For this review, take the finished solid that the model builds, in its own axes (mm). A direction names the side the tool comes from. Give positions to 0.01 mm unless a question says otherwise; leave off trailing zeros. Write each loop counter-clockwise with the first axis right and the second up, starting at its lowest first coordinate (ties: lowest second). Pieces come first, ordered by that corner, then holes.
from build123d import *

# Parameters (mm, degrees)
F0_W     = 108
F0_H     = 16
F1_DEPTH = 3
F3_D     = 2.4
F3_DEPTH = 6
F3_TIP   = 0.7210327428
F5_D     = 2.4
F5_DEPTH = 6
F5_TIP   = 0.7210327428


with BuildPart() as f1:
    # F0 (on Front) → F1 (new body, symmetric)
    with BuildSketch(Plane.XZ):
        Rectangle(F0_W, F0_H)
        with BuildLine():
            ThreePointArc((-39, -2), (-37, -4), (-39, -6))
            Line((-39, -6), (-48, -6))
            ThreePointArc((-48, -6), (-50, -4), (-48, -2))
            Line((-48, -2), (-39, -2))
        make_face(mode=Mode.SUBTRACT)
        with BuildLine():
            ThreePointArc((-39, 6), (-37, 4), (-39, 2))
            Line((-39, 2), (-48, 2))
            ThreePointArc((-48, 2), (-50, 4), (-48, 6))
            Line((-48, 6), (-39, 6))
        make_face(mode=Mode.SUBTRACT)
    extrude(amount=F1_DEPTH, both=True)

    # F3
    with Locations(Plane(origin=(0, 0, -8), x_dir=(1, 0, 0), z_dir=(0, 0, -1))):
        with Locations((36, 0), (42, 0)):
            Hole(F3_D / 2, depth=F3_DEPTH)
            with Locations((0, 0, -(F3_DEPTH + F3_TIP / 2))):  # 118° drill point
                Cone(0, F3_D / 2, F3_TIP, mode=Mode.SUBTRACT)

    # F5
    with Locations(Plane.XY.offset(8)):
        with Locations((36, 0), (42, 0)):
            Hole(F5_D / 2, depth=F5_DEPTH)
            with Locations((0, 0, -(F5_DEPTH + F5_TIP / 2))):  # 118° drill point
                Cone(0, F5_D / 2, F5_TIP, mode=Mode.SUBTRACT)


solid = f1.part
(1) The part is to be moulded in two halves that separate along Z. For faces 1 (the cylindrical face through (34.89, -0.46, 4.96)), 2 (the flat face through (-1, 0, -8)), 3 (the flat face through (-43, 0, -6)), say which applies: +Z half, -Z half, draft (parallel to the pull), parting line (faces both ways), or undercut.
(2) For L1, parallel to Y at x = 36, z = -4.65; L2, parallel to Z at x = -38, y = -0.35; L3, parallel to X at y = -2.1, z = -3.75, list the stretches that pass through material, from the lowest coordinate up.
(3) Tool access review of faces 4 (the flat face through (54, 0, 0)), 5 (the cylindrical face through (-50, 0, -4)), 6 (the cylindrical face through (40.89, 0.46, -4.96)): name each direction out of +Z, -Z, +X, -X, +Y, -Y from which nothing blocks a thin tool from reaching the whole face with its end or side.
(4) Clearance check with flat-ended pins moving along their axes: pin 1 Ø3 at (x, y) = (42, 0) entering from +Z; pin 2 Ø1.4 at (x, y) = (42, 0) entering from +Z. State where each tip first meets the part, or that it passes through.
(5) We need section B-B (x = -41). Write out the cut boundary in (y, z), and give its area (3 significant figures).
(6) We need section A-A (z = -4). Write out the cut boundary in (x, y).
The answers:
1. face 1: draft
1. face 2: -Z half
1. face 3: undercut
2. L1: y = -3 to -1.2, 1.2 to 3
2. L2: z = -8 to -5.73, -2.27 to 2.27, 5.73 to 8
2. L3: x = -54 to -49.98, -37.02 to 54
3. face 4: +Z, -Z, +X, +Y, -Y
3. face 5: +Y, -Y
3. face 6: -Z
4. pin 1: stops at z = 8
4. pin 2: stops at z = 1.7
5. outline: (-3, -8) - (3, -8) - (3, -6) - (-3, -6) - close; (-3, -2) - (3, -2) - (3, 2) - (-3, 2) - close; (-3, 6) - (3, 6) - (3, 8) - (-3, 8) - close
5. area: 48.0 mm2
6. outline: (-54, -3) - (-50, -3) - (-50, 3) - (-54, 3) - close; (-37, -3) - (54, -3) - (54, 3) - (-37, 3) - close; hole circle Ø2.4 at (36, 0); hole circle Ø2.4 at (42, 0)
